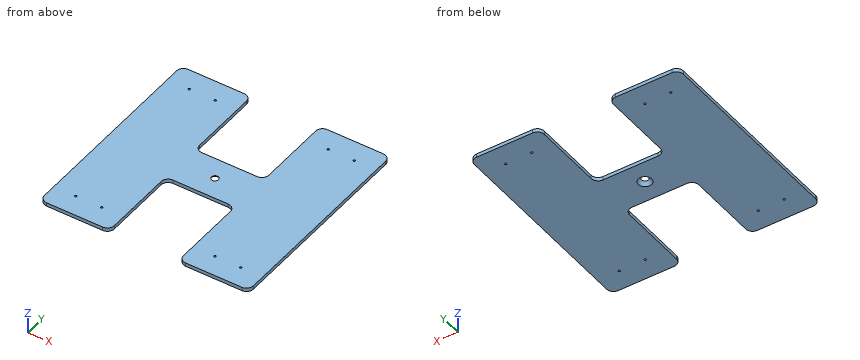
Autodesk Fusion 360 part; units mm, degrees
sketch "Sketch1" plane through (0, 0, 0) normal (0, 0, 1) x (1, 0, 0)
  line L0 (40, 31) -> (-40, 31)
  line L1 (-40, -31) -> (40, -31)
  line L2 (50, 31) -> (-50, -31) construction
  line L3 (-50, 31) -> (50, -31) construction
  line L4 (151, 31) -> (151, 141)
  line L5 (141, 151) -> (60, 151)
  line L6 (50, 141) -> (50, 41)
  line L7 (151, -31) -> (151, -141)
  line L8 (141, -151) -> (60, -151)
  line L9 (50, -141) -> (50, -41)
  line L10 (151, -31) -> (151, 31)
  line L11 (0, 0) -> (0, 31) construction
  line L12 (-141, 151) -> (-60, 151)
  line L13 (-50, 141) -> (-50, 41)
  line L14 (-151, 31) -> (-151, 141)
  line L15 (-151, -31) -> (-151, 31)
  line L16 (-141, -151) -> (-60, -151)
  line L17 (-50, -141) -> (-50, -41)
  line L18 (-151, -31) -> (-151, -141)
  circle A0 centre (0, 0) radius 5
  arc A1 (-141, 151) -> (-151, 141) centre (-141, 141) ccw
  arc A2 (-50, 141) -> (-60, 151) centre (-60, 141) ccw
  arc A3 (60, 151) -> (50, 141) centre (60, 141) ccw
  arc A4 (151, 141) -> (141, 151) centre (141, 141) ccw
  arc A5 (-151, -141) -> (-141, -151) centre (-141, -141) ccw
  arc A6 (-60, -151) -> (-50, -141) centre (-60, -141) ccw
  arc A7 (50, -141) -> (60, -151) centre (60, -141) ccw
  arc A8 (141, -151) -> (151, -141) centre (141, -141) ccw
  arc A9 (-40, -31) -> (-50, -41) centre (-40, -41) ccw
  arc A10 (50, -41) -> (40, -31) centre (40, -41) ccw
  arc A11 (40, 31) -> (50, 41) centre (40, 41) ccw
  arc A12 (-50, 41) -> (-40, 31) centre (-40, 41) ccw
  line L19 (100.5, -151) -> (100.5, -121) construction
  line L20 (119.25, -121) -> (81.75, -121) construction
  circle A13 centre (119.25, -121) radius 1.5
  circle A14 centre (81.75, -121) radius 1.5
  line L21 (151, 0) -> (100, 0) construction
  circle A15 centre (81.75, 121) radius 1.5
  circle A16 centre (119.25, 121) radius 1.5
  line L22 (0, -150) -> (0, -125) construction
  circle A17 centre (-81.75, -121) radius 1.5
  circle A18 centre (-119.25, -121) radius 1.5
  circle A19 centre (-81.75, 121) radius 1.5
  circle A20 centre (-119.25, 121) radius 1.5
  point P0 (50, 151)
  point P1 (50, -151)
  dimension "d1" = 100
  dimension "d2" = 62
  dimension "d3" = 101
  dimension "d4" = 120
  dimension "d5" = 101
  dimension "d6" = 120
  dimension "d9" = 10
  dimension "d10" = 10
  dimension "d11" = 30
  dimension "d12" = 18.75
  dimension "d13" = 37.5
  dimension "d14" = 3
  dimension "d15" = 3
  dimension "d21" = 51
  dimension "d22" = 25
  dimension "d23" = 125
extrude "Extrude1" add sketch "Sketch1" along normal blind 30.6
chamfer "Chamfer1" distance 5.2024 angle 41 1 edges at (-4.6616, 1.8081, 0) measured on face at (4.9938, -0.2492, 20.4)
extrude "Extrude2" cut 1 faces at (-96.5316, 12.7276, 30.6) along direction (0, 0, -1) blind 25.4
equation "d7 = 5.2 mm + 1 in"
equation "d12 = ( 37.5 / 2 ) * 1 mm"
The model under review builds one solid part; all positions refer to its coordinate system, in mm. Round coordinates to 2 decimals unless told otherwise and drop trailing zeros. Write each loop counter-clockwise with the first axis right and the second up, starting at its lowest first coordinate (ties: lowest second). Pieces come first, ordered by that corner, then holes. Notation, with made-up numbers: (55, -36.75) - (100, -36.75) arc R20 cw to (100, -31.75) - close; hole circle Ø5 at (-6, 78.25). An arc over 180 degrees is marked (long way). Use one line per item in the form item = value.
Q1. Consider section A-A (y = 107.5). State the section outline as (x, z) points.
Answer key:
outline = (-151, 0) - (-50, 0) - (-50, 5.2) - (-151, 5.2) - close; (50, 0) - (151, 0) - (151, 5.2) - (50, 5.2) - close
Q2. Consider section B-B (z = 2.15). State how many separate pieces and enclosed holes the cut face has, and give its area (3 significant figures).
Answer key:
separate_pieces = 1
enclosed_holes = 9
area = 66,900 mm2
Q3. Insertion check: pin 1 Ø1.5 at (x, z) = (58.5, 1.5) entering from -Y; pin 2 Ø2.5 at (x, z) = (6, 3) entering from -Y; pin 3 Ø2.5 at (x, y) = (119.25, -121) entering from +Z. Each pin has a flat end and moves straight along its axis. Give the tip position at first contact, or say it passes through.
Answer key:
pin_1 = -150.97
pin_2 = -31
pin_3 = through
Q4. Consider section C-C (x = 0). State the section outline as (y, z) points.
Answer key:
outline = (-31, 0) - (-9.52, 0) - (-5, 5.2) - (-31, 5.2) - close; (5, 5.2) - (9.52, 0) - (31, 0) - (31, 5.2) - close
Q5. Consider section D-D (x = -35). State the section outline as (y, z) points.
Answer key:
outline = (-31, 0) - (31, 0) - (31, 5.2) - (-31, 5.2) - close
Q6. For line 1 (X direction, y = 121, z = 3.3); line 2 (Y direction, x = -119.25, z = 3.9); line 3 (X direction, y = -115.5, z = 3.1), list the stretches that pass through material, from the lowest coordinate up. Write a range as [from, to].
Answer key:
line_1 = [-151, -120.75], [-117.75, -83.25], [-80.25, -50], [50, 80.25], [83.25, 117.75], [120.75, 151]
line_2 = [-151, -122.5], [-119.5, 119.5], [122.5, 151]
line_3 = [-151, -50], [50, 151]
